from build123d import *

# Parameters (mm, degrees)
SKETCH1_R           = 45
BOSS_EXTRUDE1_DEPTH = 30
SKETCH2_R           = 4
CUT_EXTRUDE1_DEPTH  = 20
SKETCH4_R           = 2.5
CUT_EXTRUDE2_DEPTH  = 30
SKETCH5_W           = 45
SKETCH5_H           = 45
CUT_EXTRUDE3_DEPTH  = 20
SKETCH6_R           = 12.5
CUT_EXTRUDE4_DEPTH  = 10


with BuildPart() as part:
    # Sketch1 → Boss-Extrude1 (new body)
    with BuildSketch(Plane(origin=(0, 0, 0), x_dir=(1, 0, 0), z_dir=(0, 1, 0))):
        Circle(SKETCH1_R)
    extrude(amount=BOSS_EXTRUDE1_DEPTH)

    # Sketch2 → Cut-Extrude1 (cut)
    with BuildSketch(Plane.XZ):
        with Locations((0, 32.5)):
            Circle(SKETCH2_R)
        with Locations((0, -32.5)):
            Circle(SKETCH2_R)
    extrude(amount=-CUT_EXTRUDE1_DEPTH, mode=Mode.SUBTRACT)

    # Sketch4 → Cut-Extrude2 (cut)
    with BuildSketch(Plane(origin=(0, 0, 0), x_dir=(-1, 0, 0), z_dir=(0, -1, 0))):
        with Locations((-30, 0)):
            Circle(SKETCH4_R)
        with Locations((-15, 25.980762114)):
            Circle(SKETCH4_R)
        with Locations((15, 25.980762114)):
            Circle(SKETCH4_R)
        with Locations((30, 0)):
            Circle(SKETCH4_R)
        with Locations((15, -25.980762114)):
            Circle(SKETCH4_R)
        with Locations((-15, -25.980762114)):
            Circle(SKETCH4_R)
    extrude(amount=-CUT_EXTRUDE2_DEPTH, mode=Mode.SUBTRACT)

    # Sketch5 → Cut-Extrude3 (cut)
    with BuildSketch(Plane(origin=(0, 0, 0), x_dir=(-1, 0, 0), z_dir=(0, -1, 0))):
        Rectangle(SKETCH5_W, SKETCH5_H)
    extrude(amount=-CUT_EXTRUDE3_DEPTH, mode=Mode.SUBTRACT)

    # Sketch6 → Cut-Extrude4 (cut)
    with BuildSketch(Plane.XZ.offset(-20)):
        with BuildLine():
            Line((-15.5, 14), (-15.5, 15.5))
            Line((-15.5, 15.5), (-14, 15.5))
            ThreePointArc((-14, 15.5), (-16.560660172, 16.560660172), (-15.5, 14))
        make_face()
        with BuildLine():
            Line((-14, 15.5), (-15.5, 15.5))
            Line((-15.5, 15.5), (-15.5, 14))
            ThreePointArc((-15.5, 14), (-14.439339828, 14.439339828), (-14, 15.5))
        make_face()
        with BuildLine():
            ThreePointArc((17, 15.5), (15.5, 17), (14, 15.5))
            Line((14, 15.5), (15.5, 15.5))
            Line((15.5, 15.5), (15.5, 14))
            ThreePointArc((15.5, 14), (16.560660172, 14.439339828), (17, 15.5))
        make_face()
        with BuildLine():
            Line((15.5, 15.5), (14, 15.5))
            ThreePointArc((14, 15.5), (14.439339828, 14.439339828), (15.5, 14))
            Line((15.5, 14), (15.5, 15.5))
        make_face()
        Circle(SKETCH6_R)
        with BuildLine():
            ThreePointArc((17, -15.5), (16.560660172, -14.439339828), (15.5, -14))
            Line((15.5, -14), (15.5, -15.5))
            Line((15.5, -15.5), (14, -15.5))
            ThreePointArc((14, -15.5), (15.5, -17), (17, -15.5))
        make_face()
        with BuildLine():
            Line((15.5, -15.5), (15.5, -14))
            ThreePointArc((15.5, -14), (14.439339828, -14.439339828), (14, -15.5))
            Line((14, -15.5), (15.5, -15.5))
        make_face()
        with BuildLine():
            ThreePointArc((-14, -15.5), (-14.439339828, -14.439339828), (-15.5, -14))
            Line((-15.5, -14), (-15.5, -15.5))
            Line((-15.5, -15.5), (-14, -15.5))
        make_face()
        with BuildLine():
            Line((-15.5, -15.5), (-15.5, -14))
            ThreePointArc((-15.5, -14), (-16.560660172, -16.560660172), (-14, -15.5))
            Line((-14, -15.5), (-15.5, -15.5))
        make_face()
    extrude(amount=-CUT_EXTRUDE4_DEPTH, mode=Mode.SUBTRACT)


solid = part.part
Build history of the part. All positions in model axes, mm. A direction names the side the tool comes from. Give positions to 0.01 mm unless a question says otherwise; leave off trailing zeros. Order: outer loops, then holes, each group sorted by start corner. A loop starts at its lowest first (then second) coordinate and runs counter-clockwise, first axis right, second up. Notation, with made-up numbers: M -33.75,-40 L -13.75,-40 A6 ccw -13.75,-30 Z; hole C 77.25,73.5 d10. An arc over 180 degrees is marked long. Put each result on its own line as item: value.
Item 1: Cut at C-C on y = 15.75. Count the separate pieces of the cut face and the enclosed holes in it, then the cut area to 3 significant figures.
Results are:
separate pieces: 1
enclosed holes: 9
area: 4,120 mm2
Item 2: Cut at A-A on z = 0. Write the cut outline in (x, y), then the cut area to 3 significant figures.
Results are:
outline: M -45,0 L -32.5,0 L -32.5,30 L -45,30 Z; M -27.5,0 L -22.5,0 L -22.5,20 L -12.5,20 L -12.5,30 L -27.5,30 Z; M 12.5,20 L 22.5,20 L 22.5,0 L 27.5,0 L 27.5,30 L 12.5,30 Z; M 32.5,0 L 45,0 L 45,30 L 32.5,30 Z
area: 1,250 mm2
Item 3: Which spindle directions (+Z, -Z, +X, -X, +Y, -Y) get a long thin tool onto all of the face, cutting with end or side? Do faces 1 (the face through (10, 20, -10)), 2 (the face through (-12.5, 14.8, 25.9)). Say none if no direction does.
Results are:
face 1: -Y
face 2: +Y, -Y
Item 4: Pull direction Z, two halves, no side cores. Call faces 3 (the face through (-27.5, 14.8, -0.1)), 4 (the face through (17.498, 14.79, -26.091)), 5 (the face through (20.765, 14.79, 39.923)), 6 (the face through (9, 0, 29)): +Z half, -Z half, draft (parallel to the pull), parting line (faces both ways), or undercut.
Results are:
face 3: undercut
face 4: undercut
face 5: parting line
face 6: draft
Item 5: Cut at B-B on x = 0. Write the cut outline in (y, z).
Results are:
outline: M 0,-45 L 30,-45 L 30,-12.5 L 20,-12.5 L 20,-22.5 L 0,-22.5 L 0,-28.5 L 20,-28.5 L 20,-36.5 L 0,-36.5 Z; M 0,22.5 L 20,22.5 L 20,12.5 L 30,12.5 L 30,45 L 0,45 L 0,36.5 L 20,36.5 L 20,28.5 L 0,28.5 Z
Item 6: Wall check: probe 1 along Z at (x, y) = (0, 14); probe 2 along X at (y, z) = (17, 0); probe 3 along X at (y, z) = (26.75, 0.5). Give the ranges that are in metal, low to high.
Results are:
probe 1: -45 to -36.5, -28.5 to -22.5, 22.5 to 28.5, 36.5 to 45
probe 2: -45 to -32.5, -27.5 to -22.5, 22.5 to 27.5, 32.5 to 45
probe 3: -45 to -32.45, -27.55 to -12.49, 12.49 to 27.55, 32.45 to 45
Item 7: Drop flat-ended pins along their axis: pin 1 Ø8 at (x, y) = (10.5, 23.5) entering from -Z; pin 2 Ø1 at (y, z) = (13, 20) entering from -X; pin 3 Ø12 at (y, z) = (18.5, -2) entering from -X; pin 4 Ø4 at (x, z) = (-15.5, 15.5) entering from -Y. Give the stop position or say it passes through.
Results are:
pin 1: z = -44.53
pin 2: x = -40.56
pin 3: x = -45
pin 4: y = 20
